```python
from build123d import *

# Parameters (mm, degrees)
CROQUIS3_R              = 11.401652729
CROQUIS3_R_2            = 11.401667337
CROQUIS3_R_3            = 11.897340247
CROQUIS3_R_4            = 11.897352739
SALIENTE_EXTRUIR3_DEPTH = 190
ESCALA1_SCALE           = 0.1
CORTAR_EXTRUIR1_REACH   = 445.395
CROQUIS4_R              = 1.5


with BuildPart() as part:
    # Croquis3 → Saliente-Extruir3 (new body)
    with BuildSketch(Plane.XY):
        Polygon((62.000007629, 600), (62.000007629, 225.000019073), (74.00001049, 225.000019073), (74.00001049, 214.000015259), (87.000007629, 214.000015259), (87.000007629, 178.000011444), (74.00001049, 178.000011444), (74.00001049, 167.000007629), (62.000007629, 167.000007629), (62.000007629, 5.000014305), (65.960402489, 2.275037766), (70.457281385, 0.575536435), (75.230016146, 1.277e-05), (698.796314631, 1.277e-05), (703.5598034, 0.579722678), (708.047413263, 2.279101392), (712.000045776, 5.000014305), (712.000045776, 167.000007629), (700, 167.000007629), (700, 178.000011444), (687.000045776, 178.000011444), (687.000045776, 214.000015259), (700, 214.000015259), (700, 225.000019073), (712.000045776, 225.000019073), (712.000045776, 600), (774.000005259, 600), (774.000005259, 752.00002538), (694.509434327, 752.00002538), (690.625557849, 752.509989697), (687.005212426, 754.008120277), (683.896969683, 756.390727503), (681.511844529, 759.497038521), (680.011611015, 763.116513016), (679.499106553, 767.000055121), (678.047678684, 777.998361779), (673.800452258, 788.246775122), (667.046530749, 797.047511795), (658.245794076, 803.801433304), (647.997385964, 808.04865973), (636.999123424, 809.500087598), (626.000816766, 808.04865973), (615.752403424, 803.801433304), (606.95162999, 797.047511795), (600.197708482, 788.246775122), (595.950463171, 777.998361779), (594.499035302, 767.000055121), (593.986767843, 763.118308924), (592.487747317, 759.501223225), (590.103931003, 756.3950759), (586.997742405, 754.011313366), (583.380656707, 752.512292839), (579.49891051, 752.00002538), (548.999055228, 752.00002538), (548.999055228, 639.999074709), (548.147197279, 633.528619953), (545.649669298, 627.49905312), (541.676700243, 622.321402668), (536.499049791, 618.348433613), (530.469542427, 615.850917196), (523.99905113, 614.999054437), (517.528559834, 615.850917196), (511.499052469, 618.348433613), (506.321327187, 622.321402668), (502.348358132, 627.49905312), (499.850909117, 633.528619953), (498.999051168, 639.999074709), (498.999051168, 752.00002538), (446.998930409, 752.00002538), (446.998930409, 707.189762429), (446.168386872, 700.691496039), (443.684287831, 694.629639501), (439.715890971, 689.4172413), (434.533657196, 685.409524601), (428.490716264, 682.879616244), (421.998901713, 682.000023228), (352.188721049, 682.000023228), (345.690420663, 682.830483045), (339.628518676, 685.314615834), (334.416116333, 689.283045399), (330.408433532, 694.465235341), (327.878564453, 700.508173573), (326.998895263, 707.00002538), (326.998895263, 752.00002538), (274.999042406, 752.00002538), (274.999042406, 639.999074709), (274.147184457, 633.528619953), (271.649656477, 627.49905312), (267.676700082, 622.321402668), (262.499033131, 618.348433613), (256.469494216, 615.850917196), (249.999032319, 614.999054437), (243.528541023, 615.850917196), (237.499033658, 618.348433613), (232.321366707, 622.321402668), (228.348397652, 627.49905312), (225.850869671, 633.528619953), (224.999011722, 639.999074709), (224.999011722, 752.00002538), (194.509863476, 752.00002538), (190.625986998, 752.509989697), (187.007479722, 754.008120277), (183.899236979, 756.390727503), (181.514111826, 759.497038521), (180.012558361, 763.116513016), (179.500053899, 767.000055121), (178.04862603, 777.998361779), (173.801399604, 788.246775122), (167.047478096, 797.047511795), (158.246713776, 803.801433304), (147.998300434, 808.04865973), (136.999993776, 809.500087598), (126.001687117, 808.04865973), (115.753273775, 803.801433304), (106.952500342, 797.047511795), (100.198578833, 788.246775122), (95.951352407, 777.998361779), (94.499924539, 767.000055121), (93.987657079, 763.118308924), (92.488636553, 759.501223225), (90.104895736, 756.3950759), (86.998707138, 754.011313366), (83.381621439, 752.512292839), (79.499875242, 752.00002538), (0, 752.00002538), (0, 600), align=None)
        with Locations((136.999993776, 767.000055121)):
            Circle(CROQUIS3_R, mode=Mode.SUBTRACT)
        with Locations((636.999123424, 767.000055121)):
            Circle(CROQUIS3_R_2, mode=Mode.SUBTRACT)
        with Locations((112.000007629, 137.000017166)):
            Circle(CROQUIS3_R_3, mode=Mode.SUBTRACT)
        with Locations((662.000007629, 137.000017166)):
            Circle(CROQUIS3_R_4, mode=Mode.SUBTRACT)
    extrude(amount=SALIENTE_EXTRUIR3_DEPTH)


with BuildPart() as part_1:
    # Escala1: scaled about (387.000056508, 381.051372624, 95)
    add(part.part.scale(ESCALA1_SCALE).moved(Location((348.300050857, 342.946235362, 85.5))))

    # Cortar-Extruir1: up to this face of the body (flat: up to its plane)
    cortar_extruir1_end = Plane(part_1.part.faces().sort_by_distance((425.700051383, 410.546236631, 95))[0])
    # Croquis4 → Cortar-Extruir1 (cut, up to the picked face)
    with BuildSketch(Plane.ZY.offset(-348.300050857), mode=Mode.PRIVATE) as cortar_extruir1_sk1:
        with Locations((90.5, 410.646237899)):
            Circle(CROQUIS4_R)
    cortar_extruir1_tool1 = split(extrude(cortar_extruir1_sk1.sketch, amount=-CORTAR_EXTRUIR1_REACH, mode=Mode.PRIVATE), bisect_by=cortar_extruir1_end, keep=Keep.BOTH, mode=Mode.PRIVATE)
    # Croquis4 → Cortar-Extruir1 (cut, up to the picked face)
    with BuildSketch(Plane.ZY.offset(-348.300050857), mode=Mode.PRIVATE) as cortar_extruir1_sk2:
        with Locations(Location((90.5, 359.446236792, 0), (0, 0, 7.662229932))):
            Circle(CROQUIS4_R)
    cortar_extruir1_tool2 = split(extrude(cortar_extruir1_sk2.sketch, amount=-CORTAR_EXTRUIR1_REACH, mode=Mode.PRIVATE), bisect_by=cortar_extruir1_end, keep=Keep.BOTH, mode=Mode.PRIVATE)
    add(cortar_extruir1_tool1.solids().sort_by(Axis((348.300051, 410.646238, 90.5), (1, 0, 0)))[0], mode=Mode.SUBTRACT)
    add(cortar_extruir1_tool2.solids().sort_by(Axis((348.300051, 359.446237, 90.5), (1, 0, 0)))[0], mode=Mode.SUBTRACT)


solid = part_1.part
```
Source: CAD feature listing. Evaluate the final solid. Frame: model axes, mm. A direction names the side the tool comes from. Coordinates: 2 decimals unless noted, no trailing zeros. One line per item, written item: value. Start each with the question number.
Q1. Mould query, pull axis X, two halves, no side actions, for faces 6 (the face through (357, 363, 95)), 7 (the face through (386, 384, 104.5)), 8 (the face through (419.5, 351, 95)), 9 (the face through (369, 418.146, 95)). Classes: pulls with the +X half, pulls with the -X half, needs draft (parallel to the pull), parting line crosses it, or undercut.
Q2. Line query: line 1 along X through (y, z) = (418, 89.25); line 2 along X through (y, z) = (357.5, 102.75); line 3 along Y through (x, z) = (370.5, 90.75). Output: solid intervals per line, ascending.
Q3. Section query A-A, the plane z = 87.25. Give the number of separate pieces and of enclosed holes in the cut face, and give its area (3 significant figures).
Q4. Contact query for flat-ended pins moving along their axis: P1, Ø0.6, axis at y = 360, z = 87.5, coming from the +X side; P2, Ø1.1, axis at y = 363, z = 91.5, coming from the +X side; P3, Ø10, axis at x = 356.5, z = 94, coming from the +Y side. Output: stop coordinate, or through.
Q5. Set-up query: faces 1 (the face through (396, 418.146, 95)), 2 (the face through (386, 384, 85.5)), 3 (the face through (417, 363, 95)), 4 (the face through (352, 418.146, 95)), 5 (the face through (423, 402.946, 95)). Return all of +Z, -Z, +X, -X, +Y, -Y with unobstructed straight access to the full face (end or side cutting, diameter ignored); none if empty.
Results:
1. face 6: pulls with the -X half
1. face 7: needs draft
1. face 8: pulls with the +X half
1. face 9: undercut
2. line 1: 348.3 to 370.8, 375.8 to 381, 393 to 398.2, 403.2 to 425.7
2. line 2: 354.5 to 358.67, 360.33 to 413.67, 415.33 to 419.5
2. line 3: 342.95 to 357.97, 360.93 to 409.17, 412.13 to 418.15
3. separate pieces: 1
3. enclosed holes: 4
3. area: 4,910 mm^2
4. P1: x = 418.3
4. P2: x = 417
4. P3: y = 423.83
5. face 1: +Z, -Z, +Y
5. face 2: -Z, +X, -X, +Y, -Y
5. face 3: +Z, -Z, +X
5. face 4: +Z, -Z, -X, +Y
5. face 5: +Z, -Z, +X, -Y
